Here's the drawing with two shaded views (mm, measured from the low corner). I have some questions. A direction names the side the tool comes from. Give positions to 0.01 mm unless a question says otherwise; leave off trailing zeros. Order: outer loops, then holes, each group sorted by start corner. A loop starts at its lowest first (then second) coordinate and runs counter-clockwise, first axis right, second up. Notation, with made-up numbers: M 19,63 L 74,63 A18 ccw 74,91 Z; hole C -13.75,-16.5 d4. An arc over 180 degrees is marked long. Write each question's results on one line, items separated by ' | '.
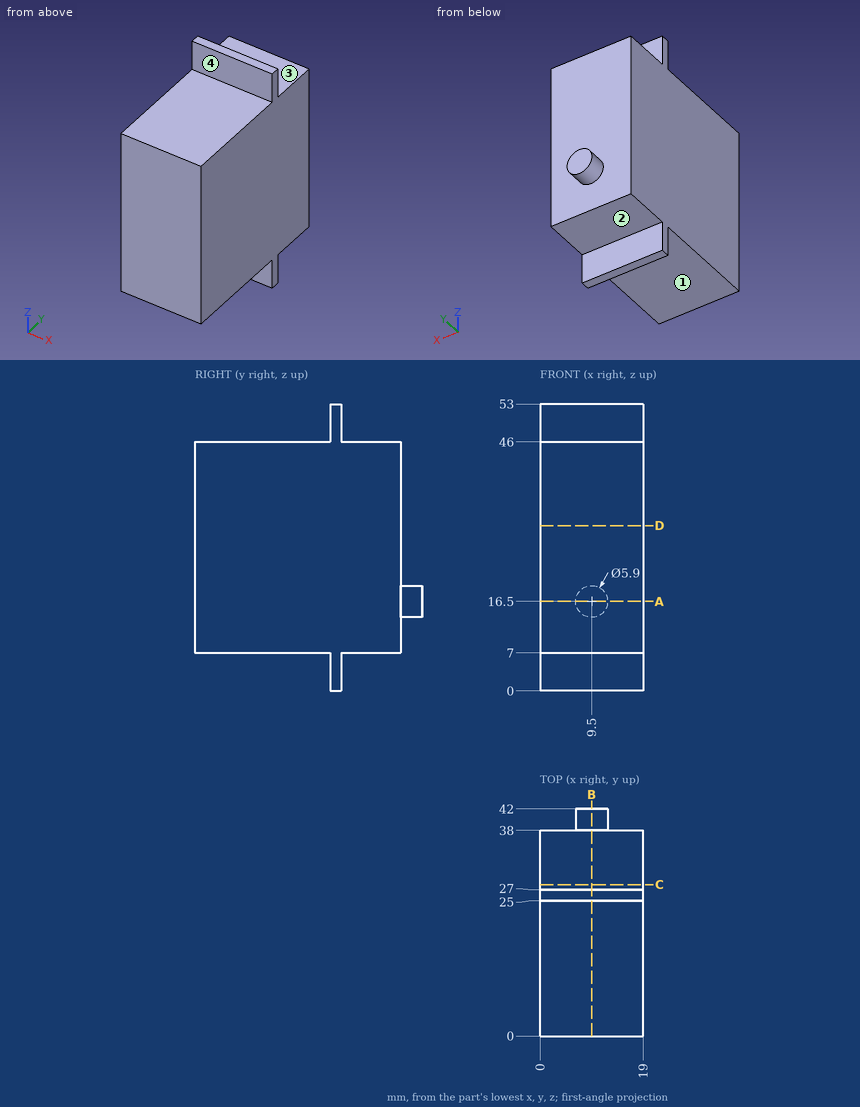
(1) Imagine slicing it at A-A, the plane z = 16.5. Write out the boundary of the cut face in (x, y).
Data:
outline: M 0,0 L 19,0 L 19,38 L 12.45,38 L 12.45,42 L 6.55,42 L 6.55,38 L 0,38 Z
(2) Will these pins go through, and if not, where does the flat tip stop? P1, Ø5, axis at x = 17, z = 34.5, coming from the -Y side; P2, Ø7.5, axis at x = 5.5, z = 49.5, coming from the +Y side; P3, Ø2, axis at x = 10, z = 3.5, coming from the -Y side; P4, Ø4, axis at x = 8, y = 30.5, coming from the +Z side.
Data:
P1: stops at y = 0 | P2: stops at y = 38 | P3: stops at y = 25 | P4: stops at z = 46
(3) For the marked faces 1, 2, 3 and 4, which set-ups out of +Z, -Z, +X, -X, +Y, -Y let a thin tool reach every point of the face, with its end or its side?
Data:
face 1: -Z, +X, -X, -Y | face 2: -Z, +X, -X, +Y | face 3: +Z, +X, -X, +Y | face 4: +Z, +X, -X, -Y
(4) Imagine slicing it at D-D, the plane z = 30.5. Write out the boundary of the cut face in (x, y).
Data:
outline: M 0,0 L 19,0 L 19,38 L 0,38 Z
(5) Imagine slicing it at B-B, the plane x = 9.5. Write out the boundary of the cut face in (y, z).
Data:
outline: M 0,7 L 25,7 L 25,0 L 27,0 L 27,7 L 38,7 L 38,13.55 L 42,13.55 L 42,19.45 L 38,19.45 L 38,46 L 27,46 L 27,53 L 25,53 L 25,46 L 0,46 Z
(6) Imagine slicing it at C-C, the plane y = 28. Write out the boundary of the cut face in (x, z).
Data:
outline: M 0,7 L 19,7 L 19,46 L 0,46 Z
(7) I need wall thicknesses on L1, parallel to Z at x = 1.75, y = 13; L2, parallel to Y at x = 5.25, z = 10; L3, parallel to Y at x = 18.25, z = 50. Which ranges of each line are inside material? Lowest first, please. Write a range as from..to.
Data:
L1: z = 7..46 | L2: y = 0..38 | L3: y = 25..27
